Read the model definition and answer for the solid it produces. Units are mm, in the model's axes. Face numbers are marked on the shaded views. A direction names the side the tool comes from. Round coordinates to 2 decimals unless told otherwise and drop trailing zeros. Order: outer loops, then holes, each group sorted by start corner. A loop starts at its lowest first (then second) coordinate and runs counter-clockwise, first axis right, second up. Notation, with made-up numbers: (-25.75, -38) - (31.25, -38) arc R13 ccw to (31.25, -24) - close; hole circle Ø2 at (-2.5, 29). An arc over 180 degrees is marked (long way). Put each result on its own line as item: value. Start each with the question number.
Q1. Section B-B on y = 16 is taken. Give the vertices of the cut face in (x, z) (3 decimals), then the cut area to 3 significant figures.
Q2. Find the intervals of material crossed by line 1 along X through (y, z) = (10.5, -50.5) (3 decimals); line 2 along X through (y, z) = (5.25, -50.5) (3 decimals); line 3 along Z through (x, y) = (4, 7.75), in increasing order. Write a range as from..to.
Q3. Section D-D on z = -14 is taken. Give the vertices of the cut face in (x, y).
Q4. Section C-C on z = -5 is taken. Give the vertices of the cut face in (x, y).
Q5. Which of the six approach directions +Z, -Z, +X, -X, +Y, -Y give full straight-line access (tool end or side, diameter ignored) to the marked faces 1 and 2?
Q6. Section A-A on x = 25 is taken. Give the vertices of the cut face in (y, z) (3 decimals), then the cut area to 3 significant figures.
Q7. Each of these flat-tipped pins is pushed along its axis until it touches: pin 1 Ø1.8 at (x, z) = (34.5, -49.5) entering from +Y; pin 2 Ø14 at (x, z) = (27.5, -23) entering from +Y; pin 3 Ø9.5 at (x, z) = (18, -10.5) entering from +Y; pin 4 Ø3 at (x, z) = (15, -50.5) entering from -Y. Where does it stop, or does it pass through?
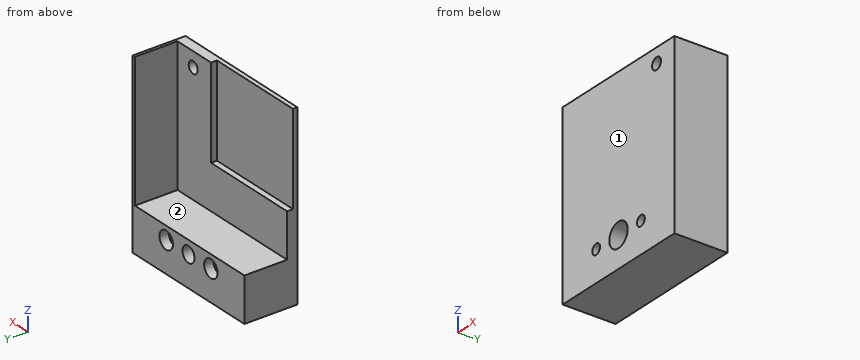
from build123d import *

# Parameters (mm, degrees)
OUTLINESKETCH2_W                               = 50
OUTLINESKETCH2_H                               = 61
OUTLINESKETCH2_R                               = 2
OUTLINEBOSS_EXTRUDE1_DEPTH                     = 18
BUILDPLATECUTOUTSKETCH1_W                      = 49
BUILDPLATECUTOUTSKETCH1_H                      = 46
BUILDPLATECUTOUTCUT_EXTRUDE7_DEPTH             = 14.5
HEATMATCUTSKETCH3_W                            = 34
HEATMATCUTSKETCH3_H                            = 31
HEATMATCUT_EXTRUDE8_DEPTH                      = 2
SKETCH1_R                                      = 1.75
SKETCH1_R_2                                    = 2.675
ZENDSTOPSWITCHMOUNTHOLESCUT_EXTRUDE1_DEPTH     = 81.901174281
SKETCH3_R                                      = 3
ZENDSTOPSWITCHMOUNTBOREHOLESCUT_EXTRUDE2_DEPTH = 3.1
SKETCH4_R                                      = 4.125
ZENDSTOPSWITCHCONNINGTOWERTBORECUT_EXTRU_DEPTH = 7.5


with BuildPart() as part:
    # OutlineSketch2 → OutlineBoss-Extrude1 (new body)
    with BuildSketch(Plane(origin=(0, 0, 0), x_dir=(1, 0, 0), z_dir=(0, 1, 0))):
        with Locations((25, 30.5)):
            Rectangle(OUTLINESKETCH2_W, OUTLINESKETCH2_H)
        with Locations(Location((42, 5, 0), (0, 0, 270))):
            Circle(OUTLINESKETCH2_R, mode=Mode.SUBTRACT)
    extrude(amount=OUTLINEBOSS_EXTRUDE1_DEPTH)

    # BuildPlateCutoutSketch1 → BuildPlateCutoutCut-Extrude7 (cut)
    with BuildSketch(Plane(origin=(0, 18, 0), x_dir=(1, 0, 0), z_dir=(0, 1, 0))):
        with Locations((24.5, 23)):
            Rectangle(BUILDPLATECUTOUTSKETCH1_W, BUILDPLATECUTOUTSKETCH1_H)
    extrude(amount=-BUILDPLATECUTOUTCUT_EXTRUDE7_DEPTH, mode=Mode.SUBTRACT)

    # HeatMatCutSketch3 → HeatMatCut-Extrude8 (cut)
    with BuildSketch(Plane(origin=(0, 3.5, 0), x_dir=(1, 0, 0), z_dir=(0, 1, 0))):
        with Locations((17, 15.5)):
            Rectangle(HEATMATCUTSKETCH3_W, HEATMATCUTSKETCH3_H)
    extrude(amount=-HEATMATCUT_EXTRUDE8_DEPTH, mode=Mode.SUBTRACT)

    # Sketch1 → ZEndStopSwitchMountHolesCut-Extrude1 (cut, through all)
    with BuildSketch(Plane(origin=(0, 18, 0), x_dir=(1, 0, 0), z_dir=(0, 1, 0))):
        with Locations(Location((35, 50.5, 0), (0, 0, 270))):
            Circle(SKETCH1_R)
        with Locations(Location((25, 50.5, 0), (0, 0, 270))):
            Circle(SKETCH1_R_2)
        with Locations(Location((15, 50.5, 0), (0, 0, 270))):
            Circle(SKETCH1_R)
    extrude(amount=-ZENDSTOPSWITCHMOUNTHOLESCUT_EXTRUDE1_DEPTH, mode=Mode.SUBTRACT)

    # Sketch3 → ZEndStopSwitchMountBoreHolesCut-Extrude2 (cut)
    with BuildSketch(Plane(origin=(0, 18, 0), x_dir=(1, 0, 0), z_dir=(0, 1, 0))):
        with Locations(Location((35, 50.5, 0), (0, 0, 270))):
            Circle(SKETCH3_R)
        with Locations(Location((15, 50.5, 0), (0, 0, 270))):
            Circle(SKETCH3_R)
    extrude(amount=-ZENDSTOPSWITCHMOUNTBOREHOLESCUT_EXTRUDE2_DEPTH, mode=Mode.SUBTRACT)

    # Sketch4 → ZEndStopSwitchConningTowertBoreCut-Extrude1 (cut)
    with BuildSketch(Plane.XZ):
        with Locations(Location((25, -50.5, 0), (0, 0, 270))):
            Circle(SKETCH4_R)
    extrude(amount=-ZENDSTOPSWITCHCONNINGTOWERTBORECUT_EXTRU_DEPTH, mode=Mode.SUBTRACT)


solid = part.part
Findings:
1. outline: (0, -61) - (50, -61) - (50, 0) - (49, 0) - (49, -46) - (0, -46) - close; hole circle Ø6 at (15, -50.5); hole circle Ø5.35 at (25, -50.5); hole circle Ø6 at (35, -50.5)
1. area: 717 mm2
2. line 1: 0..13.25, 16.75..22.325, 27.675..33.25, 36.75..50
2. line 2: 0..13.25, 16.75..20.875, 29.125..33.25, 36.75..50
2. line 3: -61..-46
3. outline: (0, 0) - (50, 0) - (50, 18) - (49, 18) - (49, 3.5) - (34, 3.5) - (34, 1.5) - (0, 1.5) - close
4. outline: (0, 0) - (40, 0) - (40, 3.5) - (34, 3.5) - (34, 1.5) - (0, 1.5) - close; (44, 0) - (50, 0) - (50, 18) - (49, 18) - (49, 3.5) - (44, 3.5) - close
5. face 1: +Z, -Z, +X, -X, -Y
5. face 2: +Z, -X, +Y
6. outline: (0, -61) - (18, -61) - (18, -53.175) - (7.5, -53.175) - (7.5, -54.625) - (0, -54.625) - close; (0, -46.375) - (7.5, -46.375) - (7.5, -47.825) - (18, -47.825) - (18, -46) - (3.5, -46) - (3.5, -31) - (1.5, -31) - (1.5, 0) - (0, 0) - close
6. area: 251 mm2
7. pin 1: y = 14.9
7. pin 2: y = 3.5
7. pin 3: y = 1.5
7. pin 4: through
